Here's how the part is built. I have some questions about the finished solid (model axes, mm). A direction names the side the tool comes from. Round coordinates to 2 decimals unless told otherwise and drop trailing zeros. Write each loop counter-clockwise with the first axis right and the second up, starting at its lowest first coordinate (ties: lowest second). Pieces come first, ordered by that corner, then holes. Notation, with made-up numbers: (-11.5, 76) -> (32.5, 76) arc R32 ccw to (32.5, 106) -> close; hole circle Ø9 at (23.5, 37). An arc over 180 degrees is marked (long way). Answer as CSV lines item,"result".
from build123d import *

# Parameters (mm, degrees)
SKETCH1_R           = 4.191
BOSS_EXTRUDE1_DEPTH = 2.921


with BuildPart() as part:
    # Sketch1 → Boss-Extrude1 (new body)
    with BuildSketch(Plane.XY):
        with BuildLine():
            Line((8.037087805, 10.932568983), (8.977813448, 11.137211321))
            ThreePointArc((8.977813448, 11.137211321), (9.528628972, 10.996624041), (9.746174499, 10.471422679))
            Line((9.746174499, 10.471422679), (9.677494343, 9.511148627))
            ThreePointArc((9.677494343, 9.511148627), (9.521666859, 8.798964182), (9.169962135, 8.160377715))
            ThreePointArc((9.169962135, 8.160377715), (9.081331887, 5.836217624), (11.232280603, 4.95134754))
            ThreePointArc((11.232280603, 4.95134754), (11.959262708, 5.005991004), (12.671821542, 4.851884559))
            Line((12.671821542, 4.851884559), (13.573848312, 4.515445968))
            ThreePointArc((13.573848312, 4.515445968), (13.961216597, 4.099383066), (13.860282246, 3.539941575))
            Line((13.860282246, 3.539941575), (13.283341474, 2.769238931))
            ThreePointArc((13.283341474, 2.769238931), (12.767215072, 2.254357949), (12.126096321, 1.907290757))
            ThreePointArc((12.126096321, 1.907290757), (10.218805564, 0), (12.126096321, -1.907290757))
            ThreePointArc((12.126096321, -1.907290757), (12.767215072, -2.254357949), (13.283341474, -2.769238931))
            Line((13.283341474, -2.769238931), (13.860282246, -3.539941575))
            ThreePointArc((13.860282246, -3.539941575), (13.961216597, -4.099383066), (13.573848312, -4.515445968))
            Line((13.573848312, -4.515445968), (12.671821542, -4.851884559))
            ThreePointArc((12.671821542, -4.851884559), (11.959262708, -5.005991004), (11.232280603, -4.95134754))
            ThreePointArc((11.232280603, -4.95134754), (8.596606282, -5.524703393), (9.169962135, -8.160377715))
            ThreePointArc((9.169962135, -8.160377715), (9.521666859, -8.798964182), (9.677494343, -9.511148627))
            Line((9.677494343, -9.511148627), (9.746174499, -10.471422679))
            ThreePointArc((9.746174499, -10.471422679), (9.528628972, -10.996624041), (8.977813448, -11.137211321))
            Line((8.977813448, -11.137211321), (8.037087805, -10.932568983))
            ThreePointArc((8.037087805, -10.932568983), (7.354328934, -10.676973184), (6.772295158, -10.237967978))
            ThreePointArc((6.772295158, -10.237967978), (4.245045246, -9.295352495), (3.302429764, -11.822602407))
            ThreePointArc((3.302429764, -11.822602407), (3.253056696, -12.549961458), (2.999111137, -13.233335836))
            Line((2.999111137, -13.233335836), (2.537725212, -14.078301071))
            ThreePointArc((2.537725212, -14.078301071), (2.070768976, -14.40251458), (1.531386247, -14.222990771))
            Line((1.531386247, -14.222990771), (0.850635478, -13.542240001))
            ThreePointArc((0.850635478, -13.542240001), (0.414447687, -12.958091818), (0.162153851, -12.27410592))
            ThreePointArc((0.162153851, -12.27410592), (-1.454287661, -10.114792857), (-3.613600724, -11.731234369))
            ThreePointArc((-3.613600724, -11.731234369), (-4.048375984, -12.316434644), (-4.631468665, -12.75403242))
            Line((-4.631468665, -12.75403242), (-5.4764339, -13.215418345))
            ThreePointArc((-5.4764339, -13.215418345), (-6.04454554, -13.235708504), (-6.401245266, -12.793071146))
            Line((-6.401245266, -12.793071146), (-6.605887604, -11.852345504))
            ThreePointArc((-6.605887604, -11.852345504), (-6.657017772, -11.125107857), (-6.499470159, -10.413301958))
            ThreePointArc((-6.499470159, -10.413301958), (-6.691894511, -7.722857955), (-9.382338515, -7.915282308))
            ThreePointArc((-9.382338515, -7.915282308), (-10.064477893, -8.172526855), (-10.79158989, -8.225413826))
            Line((-10.79158989, -8.225413826), (-11.751863943, -8.15673367))
            ThreePointArc((-11.751863943, -8.15673367), (-12.240759555, -7.866658497), (-12.301526637, -7.301441824))
            Line((-12.301526637, -7.301441824), (-11.965088046, -6.399415053))
            ThreePointArc((-11.965088046, -6.399415053), (-11.614927125, -5.759980758), (-11.097558316, -5.246348201))
            ThreePointArc((-11.097558316, -5.246348201), (-9.804872137, -2.878970219), (-12.172250119, -1.586284041))
            ThreePointArc((-12.172250119, -1.586284041), (-12.885179183, -1.433899534), (-13.525457575, -1.08528446))
            Line((-13.525457575, -1.08528446), (-14.296160219, -0.508343688))
            ThreePointArc((-14.296160219, -0.508343688), (-14.5506189, 0), (-14.296160219, 0.508343688))
            Line((-14.296160219, 0.508343688), (-13.525457575, 1.08528446))
            ThreePointArc((-13.525457575, 1.08528446), (-12.885179183, 1.433899534), (-12.172250119, 1.586284041))
            ThreePointArc((-12.172250119, 1.586284041), (-9.804872137, 2.878970219), (-11.097558316, 5.246348201))
            ThreePointArc((-11.097558316, 5.246348201), (-11.614927125, 5.759980758), (-11.965088046, 6.399415053))
            Line((-11.965088046, 6.399415053), (-12.301526637, 7.301441824))
            ThreePointArc((-12.301526637, 7.301441824), (-12.240759555, 7.866658497), (-11.751863943, 8.15673367))
            Line((-11.751863943, 8.15673367), (-10.79158989, 8.225413826))
            ThreePointArc((-10.79158989, 8.225413826), (-10.064477893, 8.172526855), (-9.382338515, 7.915282308))
            ThreePointArc((-9.382338515, 7.915282308), (-6.691894511, 7.722857955), (-6.499470159, 10.413301958))
            ThreePointArc((-6.499470159, 10.413301958), (-6.657017772, 11.125107857), (-6.605887604, 11.852345504))
            Line((-6.605887604, 11.852345504), (-6.401245266, 12.793071146))
            ThreePointArc((-6.401245266, 12.793071146), (-6.04454554, 13.235708504), (-5.4764339, 13.215418345))
            Line((-5.4764339, 13.215418345), (-4.631468665, 12.75403242))
            ThreePointArc((-4.631468665, 12.75403242), (-4.048375984, 12.316434644), (-3.613600724, 11.731234369))
            ThreePointArc((-3.613600724, 11.731234369), (-1.454287661, 10.114792857), (0.162153851, 12.27410592))
            ThreePointArc((0.162153851, 12.27410592), (0.414447687, 12.958091818), (0.850635478, 13.542240001))
            Line((0.850635478, 13.542240001), (1.531386247, 14.222990771))
            ThreePointArc((1.531386247, 14.222990771), (2.070768976, 14.40251458), (2.537725212, 14.078301071))
            Line((2.537725212, 14.078301071), (2.999111137, 13.233335836))
            ThreePointArc((2.999111137, 13.233335836), (3.253056696, 12.549961458), (3.302429764, 11.822602407))
            ThreePointArc((3.302429764, 11.822602407), (4.245045246, 9.295352495), (6.772295158, 10.237967978))
            ThreePointArc((6.772295158, 10.237967978), (7.354328934, 10.676973184), (8.037087805, 10.932568983))
        make_face()
        Circle(SKETCH1_R, mode=Mode.SUBTRACT)
    extrude(amount=BOSS_EXTRUDE1_DEPTH)


solid = part.part
Item 1: Suppose I cut it at B-B, the plane x = -8. List the corners of the cut face in (y, z) for me.
Results found:
outline,"(-7.26, 0) -> (7.26, 0) -> (7.26, 2.92) -> (-7.26, 2.92) -> close"
Item 2: For faces 1 (the cylindrical face through (-10.05, -8.17, 1.44)), 2 (the cylindrical face through (12.775, 2.26, 1.44)), 3 (the cylindrical face through (7.345, 10.672, 1.44)), 4 (the cylindrical face through (-11.609, 5.752, 1.44)), which set-ups out of +Z, -Z, +X, -X, +Y, -Y let a thin tool reach every point of the face, with its end or its side?
Results found:
face 1,"+Z, -Z, -Y"
face 2,"+Z, -Z, +X"
face 3,"+Z, -Z, +Y"
face 4,"+Z, -Z, -X"
Item 3: Suppose I cut it at A-A, the plane y = 0. List the corners of the cut face in (x, z) for me.
Results found:
outline,"(-14.55, 0) -> (-4.19, 0) -> (-4.19, 2.92) -> (-14.55, 2.92) -> close; (4.19, 0) -> (10.22, 0) -> (10.22, 2.92) -> (4.19, 2.92) -> close"
Item 4: I need wall thicknesses on L1, parallel to Y at x = -11, z = 1.45; L2, parallel to Y at x = 0, z = 1.15; L3, parallel to Y at x = 12, z = 1.25. Which ranges of each line are inside material? Lowest first, please.
Results found:
L1,"y = -8.21 to -5.21, -1.62 to 1.62, 5.21 to 8.21"
L2,"y = -11.19 to -4.19, 4.19 to 11.19"
L3,"y = -5 to -1.9, 1.9 to 5"
Item 5: Will this pin go through, and if not, where does the flat tip stop? pin 1 (10 mm diameter, centred on x = -1, y = 5, fed in from -Z).
Results found:
pin 1,"stops at z = 0"
Item 6: If we mould it in two halves opening along X, with no side actions, what happens to faces 5 (the cylindrical face through (2.08, -14.4, 1.44)), 6 (the cylindrical face through (0.42, -12.97, 1.44)), 7 (the cylindrical face through (3.25, 12.56, 1.44))? For each: pulls with the +X half, pulls with the -X half, needs draft (parallel to the pull), parting line crosses it, or undercut.
Results found:
face 5,"parting line crosses it"
face 6,"undercut"
face 7,"pulls with the +X half"
